Read the model definition and answer for the solid it produces. Units are mm, in the model's axes. A direction names the side the tool comes from. Coordinates: 2 decimals unless noted, no trailing zeros. Loops run counter-clockwise (first coordinate to the right, second up) from the corner with the lowest first, then second, coordinate; pieces in that order, holes last.
from build123d import *

# Parameters (mm, degrees)
IZIM1_R                     = 4
Y_KSEKLIK_EKSTR_ZYON1_DEPTH = 5
KES_EKSTR_ZYON1_DEPTH       = 5
IZIM3_R                     = 1


with BuildPart() as part:
    # Çizim1 → Yükseklik-Ekstrüzyon1 (new body)
    with BuildSketch(Plane(origin=(0, 0, 0), x_dir=(0, 0, -1), z_dir=(1, 0, 0))):
        Circle(IZIM1_R)
    extrude(amount=Y_KSEKLIK_EKSTR_ZYON1_DEPTH)

    # Çizim2 → Kes-Ekstrüzyon1 (cut)
    with BuildSketch(Plane(origin=(0, 0, 0), x_dir=(0, 0, -1), z_dir=(1, 0, 0))):
        with BuildLine():
            Line((0, 3), (0, 4))
            ThreePointArc((0, 4), (0.780361288, 3.923141122), (1.530733729, 3.69551813))
            Line((1.530733729, 3.69551813), (1.148050297, 2.771638598))
            ThreePointArc((1.148050297, 2.771638598), (0.585270966, 2.942355841), (0, 3))
        make_face()
        with BuildLine():
            Line((2.121320344, 2.121320344), (2.828427125, 2.828427125))
            ThreePointArc((2.828427125, 2.828427125), (3.325878449, 2.222280932), (3.69551813, 1.530733729))
            Line((3.69551813, 1.530733729), (2.771638598, 1.148050297))
            ThreePointArc((2.771638598, 1.148050297), (2.494408837, 1.666710699), (2.121320344, 2.121320344))
        make_face()
        with BuildLine():
            Line((3, 0), (4, 0))
            ThreePointArc((4, 0), (3.923141122, -0.780361288), (3.69551813, -1.530733729))
            Line((3.69551813, -1.530733729), (2.771638598, -1.148050297))
            ThreePointArc((2.771638598, -1.148050297), (2.942355841, -0.585270966), (3, 0))
        make_face()
        with BuildLine():
            Line((2.121320344, -2.121320344), (2.828427125, -2.828427125))
            ThreePointArc((2.828427125, -2.828427125), (2.222280932, -3.325878449), (1.530733729, -3.69551813))
            Line((1.530733729, -3.69551813), (1.148050297, -2.771638598))
            ThreePointArc((1.148050297, -2.771638598), (1.666710699, -2.494408837), (2.121320344, -2.121320344))
        make_face()
        with BuildLine():
            Line((0, -3), (0, -4))
            ThreePointArc((0, -4), (-0.780361288, -3.923141122), (-1.530733729, -3.69551813))
            Line((-1.530733729, -3.69551813), (-1.148050297, -2.771638598))
            ThreePointArc((-1.148050297, -2.771638598), (-0.585270966, -2.942355841), (0, -3))
        make_face()
        with BuildLine():
            Line((-2.121320344, -2.121320344), (-2.828427125, -2.828427125))
            ThreePointArc((-2.828427125, -2.828427125), (-3.325878449, -2.222280932), (-3.69551813, -1.530733729))
            Line((-3.69551813, -1.530733729), (-2.771638598, -1.148050297))
            ThreePointArc((-2.771638598, -1.148050297), (-2.494408837, -1.666710699), (-2.121320344, -2.121320344))
        make_face()
        with BuildLine():
            Line((-3, 0), (-4, 0))
            ThreePointArc((-4, 0), (-3.923141122, 0.780361288), (-3.69551813, 1.530733729))
            Line((-3.69551813, 1.530733729), (-2.771638598, 1.148050297))
            ThreePointArc((-2.771638598, 1.148050297), (-2.942355841, 0.585270966), (-3, 0))
        make_face()
        with BuildLine():
            Line((-2.121320344, 2.121320344), (-2.828427125, 2.828427125))
            ThreePointArc((-2.828427125, 2.828427125), (-2.222280932, 3.325878449), (-1.530733729, 3.69551813))
            Line((-1.530733729, 3.69551813), (-1.148050297, 2.771638598))
            ThreePointArc((-1.148050297, 2.771638598), (-1.666710699, 2.494408837), (-2.121320344, 2.121320344))
        make_face()
    extrude(amount=KES_EKSTR_ZYON1_DEPTH, mode=Mode.SUBTRACT)

    # Süpür1: sweep along a path in Çizim4
    with BuildLine(Plane.XY) as s_p_r1_path:
        Line((5, 0), (105, 0))
        Line((105, 0), (105, 10))
    # Çizim3 → Süpür1 (sweep)
    with BuildSketch(Plane(origin=(5, 0, 0), x_dir=(0, 0, -1), z_dir=(1, 0, 0))):
        Circle(IZIM3_R)
    sweep(path=s_p_r1_path.line, transition=Transition.RIGHT)


solid = part.part
Item 1: Find the intervals of material crossed by line 1 along X through (y, z) = (2.25, -1.25); line 2 along Z through (x, y) = (93, 0.25); line 3 along Y through (x, z) = (49.5, -0.5), in increasing order.
Numbers:
line 1: x = 0 to 5
line 2: z = -0.97 to 0.97
line 3: y = -0.87 to 0.87
Item 2: A cutting plane is placed at B-B on x = 105. Determine the outline of the cut face in (y, z), then the cut area to 3 significant figures.
Numbers:
outline: (0, -1) - (10, -1) - (10, 1) - (0, 1) arc R1 ccw to start
area: 21.6 mm2
Item 3: A cutting plane is placed at A-A on x = 57. Determine the outline of the cut face in (y, z), then the cut area to 3 significant figures.
Numbers:
outline: circle Ø2 at (0, 0)
area: 3.14 mm2
Item 4: Which of the six approach directions +Z, -Z, +X, -X, +Y, -Y give full straight-line access (tool end or side, diameter ignored) to faces 1 (the face through (5, 1, -1)), 2 (the face through (106, 5, 0)), 3 (the face through (105, 10, 0))?
Numbers:
face 1: none
face 2: +Y
face 3: +Z, -Z, +X, -X, +Y
Item 5: Given pin 1 (5 mm diameter, centred on x = 44.5, y = -0.5, fed in from -Z); pin 2 (4 mm diameter, centred on x = 13.5, z = 0, fed in from +Y); pin 3 (0.5 mm diameter, centred on x = 2.5, y = 3.5, fed in from -Z), each flat-ended and moving along its own axis, determine where each tip first touches the part or whether it passes through.
Numbers:
pin 1: stops at z = -1
pin 2: stops at y = 1
pin 3: stops at z = -2.33
